The model under review builds one solid part; all positions refer to its coordinate system, in mm. Face numbers are marked on the shaded views. A direction names the side the tool comes from. Coordinates: 2 decimals unless noted, no trailing zeros. Loops run counter-clockwise (first coordinate to the right, second up) from the corner with the lowest first, then second, coordinate; pieces in that order, holes last. Notation, with made-up numbers: (26, 76) - (84, 76) arc R23 cw to (84, 104) - close; hole circle Ø1 at (-33, 27). An arc over 180 degrees is marked (long way). Answer in a Markdown table with one row per item. Add a question column.
(1) We need section B-B on z = 72.5. Write out the cut boundary in (x, y).
(2) Machinability: for the marked faces 1, 2 and 3, which of the approach directions +Z, -Z, +X, -X, +Y, -Y give a long, thin tool a straight path to every point of the face, cutting with its end or side? Answer none if there is none.
(3) We need section A-A on z = 47.5. Write out the cut boundary in (x, y).
(4) For line 1 along Z through (x, y) = (6.5, -4.4); line 2 along Y through (x, z) = (22, 25.5); line 3 along X through (y, z) = (4.4, 72.5), list the stretches that pass through material, from the lowest coordinate up.
(5) For P1, Ø5, axis at x = 20.5, y = 2, coming from the -Z side; P2, Ø3, axis at x = 21.5, y = -2, coming from the +Z side; P3, Ø5, axis at y = 2.5, z = 8.5, coming from the +X side, all flat-tipped, find the tip position at first contact; note any pin that passes through.
(6) We need section D-D on y = 3.25. Write out the cut boundary in (x, z), plus the area to 3 significant figures.
(7) We need section C-C on x = 10. Write out the cut boundary in (y, z).
from build123d import *

# Parameters (mm, degrees)
SKETCH_1_R          = 2.05
EXTRUDE_1_DEPTH     = 80
SKETCH_2_W          = 13.1
SKETCH_2_H          = 4.1
CUT_EXTRUDE_1_DEPTH = 95
SKETCH_4_R          = 2.6
CUT_EXTRUDE_2_DEPTH = 20
CUT_EXTRUDE_5_DEPTH = 20
FILLET_1_R          = 3


with BuildPart() as part:
    # 草图1 → 凸台-拉伸1 (new body)
    with BuildSketch(Plane.XY):
        with BuildLine():
            Line((0, 5), (22, 5))
            ThreePointArc((22, 5), (27, 0), (22, -5))
            Line((22, -5), (0, -5))
            Line((0, -5), (0, 5))
        make_face()
        with Locations(Location((22, 0, 0), (0, 0, 180))):
            Circle(SKETCH_1_R, mode=Mode.SUBTRACT)
    extrude(amount=EXTRUDE_1_DEPTH)

    # 草图2 → 切除-拉伸1 (cut)
    with BuildSketch(Plane.XY.offset(80)):
        with Locations((6.55, 0)):
            Rectangle(SKETCH_2_W, SKETCH_2_H)
    extrude(amount=-CUT_EXTRUDE_1_DEPTH, mode=Mode.SUBTRACT)

    # 草图4 → 切除-拉伸2 (cut)
    with BuildSketch(Plane(origin=(0, 5, 0), x_dir=(1, 0, 0), z_dir=(0, 1, 0))):
        with Locations((6.5, -32.5)):
            Circle(SKETCH_4_R)
        with Locations((6.5, -7.5)):
            Circle(SKETCH_4_R)
        with Locations((6.5, -72.5)):
            Circle(SKETCH_4_R)
        with Locations((6.5, -47.5)):
            Circle(SKETCH_4_R)
    extrude(amount=-CUT_EXTRUDE_2_DEPTH, mode=Mode.SUBTRACT)

    # 草图5 → 切除-拉伸5 (cut)
    with BuildSketch(Plane(origin=(0, 5, 0), x_dir=(1, 0, 0), z_dir=(0, 1, 0))):
        Polygon((22, 0), (32.496468361, 0), (32.496468361, -16), (16, -16), (16, 0), align=None)
        Polygon((16, -64), (32.496468361, -64), (32.496468361, -80), (22, -80), (16, -80), align=None)
    extrude(amount=-CUT_EXTRUDE_5_DEPTH, mode=Mode.SUBTRACT)

    # 圆角1
    fillet_1_edges = [part.edges().sort_by_distance(p)[0] for p in [
        (0, -3.525, 0),
        (0, -3.525, 80),
        (0, 3.525, 80),
        (0, 3.525, 0),
    ]]
    fillet(fillet_1_edges, radius=FILLET_1_R)


solid = part.part
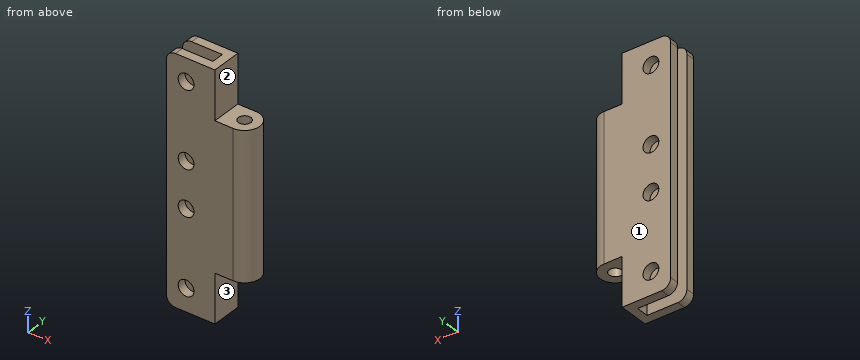
Outcome:
| question | item | result |
|---|---|---|
| 1 | outline | (0, -5) - (3.9, -5) - (3.9, -2.05) - (0, -2.05) - close; (0, 2.05) - (3.9, 2.05) - (3.9, 5) - (0, 5) - close; (9.1, -5) - (16, -5) - (16, 5) - (9.1, 5) - (9.1, 2.05) - (13.1, 2.05) - (13.1, -2.05) - (9.1, -2.05) - close |
| 2 | face 1 | +Z, -Z, +X, -X, +Y |
| 2 | face 2 | +Z, +X, +Y, -Y |
| 2 | face 3 | -Z, +X, +Y, -Y |
| 3 | outline | (0, -5) - (3.9, -5) - (3.9, -2.05) - (0, -2.05) - close; (0, 2.05) - (3.9, 2.05) - (3.9, 5) - (0, 5) - close; (9.1, -5) - (22, -5) arc R5 ccw to (22, 5) - (9.1, 5) - (9.1, 2.05) - (13.1, 2.05) - (13.1, -2.05) - (9.1, -2.05) - close; hole circle Ø4.1 at (22, 0) |
| 4 | line 1 | 0 to 4.9, 10.1 to 29.9, 35.1 to 44.9, 50.1 to 69.9, 75.1 to 80 |
| 4 | line 2 | -5 to -2.05, 2.05 to 5 |
| 4 | line 3 | 0 to 3.9, 9.1 to 16 |
| 5 | P1 | z = 16 |
| 5 | P2 | z = 64 |
| 5 | P3 | x = 16 |
| 6 | outline | (0, 3) arc R3 ccw to (3, 0) - (16, 0) - (16, 16) - (25.8, 16) - (25.8, 64) - (16, 64) - (16, 80) - (3, 80) arc R3 ccw to (0, 77) - close; hole circle Ø5.2 at (6.5, 7.5); hole circle Ø5.2 at (6.5, 32.5); hole circle Ø5.2 at (6.5, 47.5); hole circle Ø5.2 at (6.5, 72.5) |
| 6 | area | 1,660 mm² |
| 7 | outline | (-5, 0) - (-2.05, 0) - (-2.05, 80) - (-5, 80) - close; (2.05, 0) - (5, 0) - (5, 80) - (2.05, 80) - close |
